```python
from build123d import *

# Parameters (mm, degrees)
F0_W     = 50.8
F0_H     = 12.7
F1_DEPTH = 10.16
F2_W     = 51.661278
F2_H     = 9.144
F3_DEPTH = 1.27
F5_DEPTH = 59.69
F7_DEPTH = 0.508
F9_DEPTH = 0.508


with BuildPart() as f1:
    # F0 (on Top) → F1 (new body)
    with BuildSketch(Plane.XY):
        with Locations((-25.4, 6.35)):
            Rectangle(F0_W, F0_H)
    extrude(amount=F1_DEPTH)

    # F2 (on Top) → F3 (cut)
    with BuildSketch(Plane.XY):
        with Locations((-25.830639, 6.35)):
            Rectangle(F2_W, F2_H)
    extrude(amount=F3_DEPTH, mode=Mode.SUBTRACT)

    # F4 (on face) → F5 (cut)
    with BuildSketch(Plane.YZ):
        with BuildLine():
            ThreePointArc((12.619456, 10.16), (23.691939, 17.959451), (27.94, 30.819671))
            ThreePointArc((27.94, 30.819671), (-6.51022, 48.16161), (0.080544, 10.16))
            Line((0.080544, 10.16), (12.619456, 10.16))
        make_face()
        with BuildLine():
            Line((12.619456, 10.16), (0.080544, 10.16))
            ThreePointArc((0.080544, 10.16), (6.35, 9.229671), (12.619456, 10.16))
        make_face()
    extrude(amount=-F5_DEPTH, mode=Mode.SUBTRACT)

    # F6 (on face) → F7 (cut)
    with BuildSketch(Plane.YZ):
        with BuildLine():
            Line((1.778, 9.719318), (1.778, 1.27))
            Line((1.778, 1.27), (10.922, 1.27))
            Line((10.922, 1.27), (10.922, 9.719318))
            ThreePointArc((10.922, 9.719318), (6.35, 9.229671), (1.778, 9.719318))
        make_face()
    extrude(amount=-F7_DEPTH, mode=Mode.SUBTRACT)

    # F8 (on face) → F9 (cut)
    with BuildSketch(Plane(origin=(-50.8, 0, 0), x_dir=(0, -1, 0), z_dir=(-1, 0, 0))):
        with BuildLine():
            Line((-10.922, 1.27), (-1.778, 1.27))
            Line((-1.778, 1.27), (-1.778, 9.719318))
            ThreePointArc((-1.778, 9.719318), (-6.35, 9.229671), (-10.922, 9.719318))
            Line((-10.922, 9.719318), (-10.922, 1.27))
        make_face()
    extrude(amount=-F9_DEPTH, mode=Mode.SUBTRACT)


solid = f1.part
```
Geometry: final body of the model. Coordinates: model frame, mm. A direction names the side the tool comes from. Round coordinates to 2 decimals unless told otherwise and drop trailing zeros. Order: outer loops, then holes, each group sorted by start corner. A loop starts at its lowest first (then second) coordinate and runs counter-clockwise, first axis right, second up. Notation, with made-up numbers: (70, 44.25) -> (103, 44.25) arc R29 cw to (103, 70.25) -> close; hole circle Ø7 at (32, 30.25). An arc over 180 degrees is marked (long way). Use one line per item in the form item = value. Start each with the question number.
1. Draft query along Y for faces 3 (the face through (-50.292, 6, 6)), 4 (the face through (-26, 0, 5)), 5 (the face through (-26, 6, 1.27)), 6 (the face through (-26, 12, 0)). Return one class per face: pulls with the +Y half, pulls with the -Y half, needs draft (parallel to the pull), parting line crosses it, or undercut.
2. Cut plane A-A (x = -46). Return the cut outline in (y, z), then the cut area to 3 significant figures.
3. Line query: probe 1 along Y at (x, z) = (-45, 0.5); probe 2 along Z at (x, y) = (-20, 5.75); probe 3 along X at (y, z) = (2.75, 8.25). Output: solid intervals per line, ascending.
4. Cut plane C-C (y = 11.75). Return the cut outline in (x, z).
5. Reachability of faces 1 (the face through (-0.508, 6, 6)), 2 (the face through (0, 12, 5)) from +Z, -Z, +X, -X, +Y, -Y: full face, straight path, thin tool, end or side. Return the list, or none.
6. Pin query (flat end, axial travel): pin 1 Ø4 at (y, z) = (4.5, 4.5) entering from +X; pin 2 Ø3 at (x, y) = (-7.5, 5.5) entering from +Z; pin 3 Ø1 at (x, y) = (-7, 6) entering from -Z. Return the tip coordinate at first contact, or that it passes through.
7. Cut plane B-B (y = 7). Return the cut outline in (x, z).
Solution:
q1.face_3 = undercut
q1.face_4 = pulls with the -Y half
q1.face_5 = undercut
q1.face_6 = needs draft
q2.outline = (0, 0) -> (1.78, 0) -> (1.78, 1.27) -> (10.92, 1.27) -> (10.92, 0) -> (12.7, 0) -> (12.7, 10.16) -> (12.62, 10.16) arc R21.59 cw to (0.08, 10.16) -> (0, 10.16) -> close
q2.area = 110 mm^2
q3.probe_1 = 0 to 1.78, 10.92 to 12.7
q3.probe_2 = 1.27 to 9.24
q3.probe_3 = -50.29 to -0.51
q4.outline = (-50.8, 0) -> (0, 0) -> (0, 9.92) -> (-50.8, 9.92) -> close
q5.face_1 = +Z, -Z, +X
q5.face_2 = +Z, -Z, +X, +Y, -Y
q6.pin_1 = -0.51
q6.pin_2 = 9.36
q6.pin_3 = 1.27
q7.outline = (-50.29, 1.27) -> (-0.51, 1.27) -> (-0.51, 9.24) -> (-50.29, 9.24) -> close
